```python
from build123d import *

# Parameters (mm, degrees)
F0_W     = 92.643157
F0_H     = 50.231842
F1_DEPTH = 50.8
F3_DEPTH = 91.948
F4_DEPTH = 5.08
F6_DEPTH = 5.08
F9_D     = 10.16


with BuildPart() as f1:
    # F0 (on Top) → F1 (new body)
    with BuildSketch(Plane.XY):
        with Locations((0.451185, -1.203158)):
            Rectangle(F0_W, F0_H)
    extrude(amount=F1_DEPTH)

    # F2 (on face) → F3 (cut)
    with BuildSketch(Plane.XZ.offset(26.319079)):
        with BuildLine():
            Line((18.460125, 50.8), (-13.976645, 50.8))
            ThreePointArc((-13.976645, 50.8), (2.24174, 38.437578), (18.460125, 50.8))
        make_face()
    extrude(amount=-F3_DEPTH, mode=Mode.SUBTRACT)

    # F2 (on face) → F4 (join)
    with BuildSketch(Plane.XZ.offset(26.319079)):
        with BuildLine():
            ThreePointArc((18.460125, 50.8), (2.24174, 38.437578), (-13.976645, 50.8))
            Line((-13.976645, 50.8), (-20.409722, 50.8))
            ThreePointArc((-20.409722, 50.8), (2.616898, 32.474383), (25.643518, 50.8))
            Line((25.643518, 50.8), (18.460125, 50.8))
        make_face()
    extrude(amount=F4_DEPTH)

    # F5 (on face) → F6 (join)
    with BuildSketch(Plane(origin=(0, 23.912763, 0), x_dir=(-1, 0, 0), z_dir=(0, 1, 0))):
        with BuildLine():
            Line((-18.460125, 50.8), (-22.761472, 50.8))
            ThreePointArc((-22.761472, 50.8), (-2.292335, 33.518654), (18.176802, 50.8))
            Line((18.176802, 50.8), (13.976645, 50.8))
            ThreePointArc((13.976645, 50.8), (-2.24174, 38.437578), (-18.460125, 50.8))
        make_face()
    extrude(amount=F6_DEPTH)

    # F9 (through all)
    with Locations(Plane.XY.offset(50.8)):
        with Locations((-32.094348, 0), (33.174038, 0)):
            Hole(F9_D / 2)


solid = f1.part
```
Source: CAD feature listing. Evaluate the final solid. Frame: model axes, mm. A direction names the side the tool comes from. Give positions to 0.01 mm unless a question says otherwise; leave off trailing zeros. Loops run counter-clockwise (first coordinate to the right, second up) from the corner with the lowest first, then second, coordinate; pieces in that order, holes last. Notation, with made-up numbers: (63.25, -4) - (68.25, -4) arc R23 cw to (68.25, 9) - close; hole circle Ø7 at (-29, 70). An arc over 180 degrees is marked (long way). Use CSV: the item, a comma, the result in double quotes. Start each with the question number.
1. Section A-A (y = 0). Output: boundary loops of the cut face in (x, z).
2. Ray query, L1, parallel to Y at x = 33, z = 18; L2, parallel to X at y = -3, z = 32.5; L3, parallel to Y at x = -19.5, z = 47.5. Return the intervals inside material, ascending.
3. Section D-D (x = 30). Output: boundary loops of the cut face in (y, z).
4. Section B-B (z = 12). Output: boundary loops of the cut face in (x, y).
5. Reachability of faces 5 (the cylindrical face through (2.7, 26.417, 33.523)), 6 (the flat face through (2, 28.993, 38)) from +Z, -Z, +X, -X, +Y, -Y: full face, straight path, thin tool, end or side. Return the list, or none.
6. Pin query (flat end, axial travel): pin 1 (2 mm diameter, centred on x = 2.5, y = -9.5, fed in from +Z); pin 2 (3 mm diameter, centred on x = -8, z = 26, fed in from -Y). Return the tip coordinate at first contact, or that it passes through.
7. Section C-C (y = 13). Output: boundary loops of the cut face in (x, z), then the cut area to 3 significant figures.
8. Draft query along Y for faces 1 (the cylindrical face through (-36.787, -1.946, 25.044)), 2 (the flat face through (2, -31.399, 38)), 3 (the cylindrical face through (38.25, 0.22, 25.04)), 4 (the cylindrical face through (2.17, -28.82, 32.48)). Return one class per face: +Y half, -Y half, draft (parallel to the pull), parting line (faces both ways), or undercut.
Response:
1,outline,"(-45.87, 0) - (-37.17, 0) - (-37.17, 50.8) - (-45.87, 50.8) - close; (-27.01, 0) - (28.09, 0) - (28.09, 50.8) - (18.46, 50.8) arc R16.82 cw to (-13.98, 50.8) - (-27.01, 50.8) - close; (38.25, 0) - (46.77, 0) - (46.77, 50.8) - (38.25, 50.8) - close"
2,L1,"-26.32 to -5.08, 5.08 to 23.91"
2,L2,"-45.87 to -36.19, -27.99 to 29.07, 37.27 to 46.77"
2,L3,"-26.32 to 23.91"
3,outline,"(-26.32, 0) - (-3.97, 0) - (-3.97, 50.8) - (-26.32, 50.8) - close; (3.97, 0) - (23.91, 0) - (23.91, 50.8) - (3.97, 50.8) - close"
4,outline,"(-45.87, -26.32) - (46.77, -26.32) - (46.77, 23.91) - (-45.87, 23.91) - close; hole circle Ø10.16 at (-32.09, 0); hole circle Ø10.16 at (33.17, 0)"
5,face 5,"-Z, +Y"
5,face 6,"+Z, -Z, +X, -X, +Y"
6,pin 1,"z = 38.48"
6,pin 2,"y = -26.32"
7,outline,"(-45.87, 0) - (46.77, 0) - (46.77, 50.8) - (18.46, 50.8) arc R16.82 cw to (-13.98, 50.8) - (-45.87, 50.8) - close"
7,area,"4,410 mm²"
8,face 1,"undercut"
8,face 2,"-Y half"
8,face 3,"undercut"
8,face 4,"draft"
